The listing builds one solid part. Answer for the finished solid, in the listing's coordinates (mm). A direction names the side the tool comes from. Give positions to 0.01 mm unless a question says otherwise; leave off trailing zeros. Write each loop counter-clockwise with the first axis right and the second up, starting at its lowest first coordinate (ties: lowest second). Pieces come first, ordered by that corner, then holes. Notation, with made-up numbers: (52.25, 16.5) - (107.25, 16.5) arc R6 ccw to (107.25, 22.5) - close; hole circle Ø10 at (50, 85). An arc over 180 degrees is marked (long way). Return JSON: item names as keys, results as strings.
from build123d import *

# Parameters (mm, degrees)
M3X0_5_TAPPED_HOLE1_REACH           = 25.691
M3X0_5_TAPPED_HOLE1_BORE_R          = 1.25
M3X0_5_TAPPED_HOLE1_ON_FACE_2_REACH = 25.691
M3X0_5_TAPPED_HOLE1_BORE_2_R        = 1.25
CHAMFER1_SIZE                       = 0.5
BOSS_EXTRUDE1_START                 = 7.5
BOSS_EXTRUDE1_DEPTH                 = 7.5
CIRPATTERN1_COUNT                   = 20


with BuildPart() as part:
    # Sketch1 → Revolve1 (revolve)
    with BuildSketch(Plane(origin=(0, 0, 0), x_dir=(0, 0, -1), z_dir=(1, 0, 0)), mode=Mode.PRIVATE) as revolve1_sk:
        Polygon((-3.75, 7.5), (-3.75, 5.5), (3.75, 5.5), (3.75, 7.5), (4.25, 9), (4.75, 9), (4.75, 2.5), (-11.25, 2.5), (-11.25, 9), (-4.25, 9), align=None)
    revolve(revolve1_sk.sketch.rotate(Axis((0, 0, 0), (0, 0, -1)), 90), axis=Axis((0, 0, 0), (0, 0, -1)))

    # M3x0.5 Tapped Hole1 bore (on position points) → M3x0.5 Tapped Hole1 (cut, up to next)
    with BuildSketch(Plane(origin=(-9, 0, 7.75), x_dir=(0, -1, 0), z_dir=(-1, 0, 0)), mode=Mode.PRIVATE) as m3x0_5_tapped_hole1_sk1:
        Circle(M3X0_5_TAPPED_HOLE1_BORE_R)
    m3x0_5_tapped_hole1_tool1 = extrude(m3x0_5_tapped_hole1_sk1.sketch, amount=-M3X0_5_TAPPED_HOLE1_REACH, mode=Mode.PRIVATE) & part.part
    add(m3x0_5_tapped_hole1_tool1.solids().sort_by_distance((-9, 0, 7.75))[0], mode=Mode.SUBTRACT)

    # M3x0.5 Tapped Hole1 bore 2 (on position points) → M3x0.5 Tapped Hole1 on face 2 (cut, up to next)
    with BuildSketch(Plane(origin=(0, 9, 7.75), x_dir=(0, 0, 1), z_dir=(0, 1, 0)), mode=Mode.PRIVATE) as m3x0_5_tapped_hole1_on_face_2_sk1:
        Circle(M3X0_5_TAPPED_HOLE1_BORE_2_R)
    m3x0_5_tapped_hole1_on_face_2_tool1 = extrude(m3x0_5_tapped_hole1_on_face_2_sk1.sketch, amount=-M3X0_5_TAPPED_HOLE1_ON_FACE_2_REACH, mode=Mode.PRIVATE) & part.part
    add(m3x0_5_tapped_hole1_on_face_2_tool1.solids().sort_by_distance((0, 9, 7.75))[0], mode=Mode.SUBTRACT)

    # Chamfer1
    chamfer1_edges = [part.edges().sort_by_distance(p)[0] for p in [
        (-9, 0, 11.25),
    ]]
    chamfer(chamfer1_edges, length=CHAMFER1_SIZE)

    # Sketch4 → Boss-Extrude1 (add)
    with BuildSketch(Plane(origin=(0, 0, 3.75), x_dir=(-1, 0, 0), z_dir=(0, 0, -1)).offset(BOSS_EXTRUDE1_START)):
        with BuildLine():
            ThreePointArc((-0.499483204, 5.477272727), (0, 6), (0.499483204, 5.477272727))
            ThreePointArc((0.499483204, 5.477272727), (0, 5.5), (-0.499483204, 5.477272727))
        make_face()
    boss_extrude1 = extrude(amount=-BOSS_EXTRUDE1_DEPTH)

    # CirPattern1: Boss-Extrude1 ×20 about axis
    cirpattern1_axis = Axis((0, 0, 0), (0, 0, 1))
    for i in range(1, CIRPATTERN1_COUNT):
        add(boss_extrude1.rotate(cirpattern1_axis, i * 360 / CIRPATTERN1_COUNT))


solid = part.part
Item 1: Consider L1, parallel to Z at x = 3.5, y = 5.75; L2, parallel to Z at x = 0, y = 5.75; L3, parallel to Y at x = 0, z = -0.5. Determine where each line is inside the solid, lowest interval first.
Answer below:
{"L1": "z = -4.75 to -3.75, 3.75 to 11.25", "L2": "z = -4.75 to 6.5, 9 to 11.25", "L3": "y = -6 to -2.5, 2.5 to 6"}
Item 2: The mould has two halves that part along X. Classify faces 1 (the face through (-1.84, 5.71, -0.05)), 2 (the face through (-6.633, -6.083, -4.504)), 3 (the face through (-2, 2, 11.25)), 4 (the face through (3.52, -4.86, -0.05)): +X half, -X half, draft (parallel to the pull), parting line (faces both ways), or undercut.
Answer below:
{"face 1": "undercut", "face 2": "parting line", "face 3": "draft", "face 4": "undercut"}
Item 3: For faces 5 (the face through (2.385, -0.751, 3.362)), 6 (the face through (0.05, 5.63, 6.5)), 7 (the face through (-3.52, 4.86, -0.05)), determine the directions among +Z, -Z, +X, -X, +Y, -Y from which every point of the face is accessible in a straight line to the end or side of a thin tool.
Answer below:
{"face 5": "+Z, -Z", "face 6": "+Y", "face 7": "none"}
Item 4: A cutting plane is placed at A-A on z = 6.25. Determine the outline of the cut face in (x, y), then the cut area to 3 significant figures.
Answer below:
{"outline": "circle Ø18 at (0, 0); hole circle Ø5 at (0, 0)", "area": "235 mm²"}
Item 5: Flat-ended cylindrical pins translate along their axes: P1, Ø1.5, axis at x = 0, z = 7.75, coming from the +Y side; P2, Ø6, axis at y = -1.5, z = 9, coming from the -X side; P3, Ø1, axis at x = 3, z = 7.5, coming from the -Y side; P4, Ø6, axis at y = 4.5, z = 2, coming from the -X side. Find the tip coordinate at first contact, or state that the pin passes through.
Answer below:
{"P1": "stops at y = -2.38", "P2": "stops at x = -9", "P3": "stops at y = -8.65", "P4": "stops at x = -8.64"}
